from build123d import *

# Parameters (mm, degrees)
SKETCH1_R           = 1.5
BOSS_EXTRUDE1_DEPTH = 6
SKETCH2_W           = 0.5
SKETCH2_H           = 6
CUT_EXTRUDE1_DEPTH  = 0.5
FILLET1_R           = 0.5


with BuildPart() as part:
    # Sketch1 → Boss-Extrude1 (new body)
    with BuildSketch(Plane(origin=(0, 0, 0), x_dir=(1, 0, 0), z_dir=(0, 1, 0))):
        with BuildLine():
            ThreePointArc((95.828517615, 16.432423404), (96.485539703, 17.415726447), (96.511338172, 18.598053533))
            Line((96.511338172, 18.598053533), (78.7360041, 13.835167123))
            ThreePointArc((78.7360041, 13.835167123), (76.706708419, 13.046017192), (74.896318454, 11.836353292))
            Line((74.896318454, 11.836353292), (74.145485774, 11.206329867))
            ThreePointArc((74.145485774, 11.206329867), (73.602368785, 10.843430696), (72.99358008, 10.606685717))
            Line((72.99358008, 10.606685717), (44.605042506, 3))
            Line((44.605042506, 3), (0, 3))
            ThreePointArc((0, 3), (-3, 0), (0, -3))
            Line((0, -3), (44.999999999, -3))
            ThreePointArc((44.999999999, -3), (45.391578576, -2.974334584), (45.776457135, -2.897777479))
            Line((45.776457135, -2.897777479), (84.823166373, 7.564756729))
            ThreePointArc((84.823166373, 7.564756729), (85.431955077, 7.801501708), (85.975072067, 8.164400878))
            Line((85.975072067, 8.164400878), (95.828517615, 16.432423404))
        make_face()
        with Locations(Location((66.660044365, 5.803791396, 0), (0, 0, 270))):
            Circle(SKETCH1_R, mode=Mode.SUBTRACT)
        with Locations(Location((84.046709238, 10.462534208, 0), (0, 0, 270))):
            Circle(SKETCH1_R, mode=Mode.SUBTRACT)
        with Locations(Location((44.999999999, 0, 0), (0, 0, 270))):
            Circle(SKETCH1_R, mode=Mode.SUBTRACT)
        with Locations(Location((0, 0, 0), (0, 0, 270))):
            Circle(SKETCH1_R, mode=Mode.SUBTRACT)
    extrude(amount=BOSS_EXTRUDE1_DEPTH)

    # Sketch2 → Cut-Extrude1 (cut)
    with BuildSketch(Plane(origin=(1.815520398, 0, 6.775614366), x_dir=(-0.965925826289068, 0, 0.25881904510252224), z_dir=(-0.2588190451025222, 0, -0.9659258262890679))):
        with Locations((-81.167277896, 3)):
            Rectangle(SKETCH2_W, SKETCH2_H)
        with Locations((-82.567277896, 3)):
            Rectangle(SKETCH2_W, SKETCH2_H)
        with Locations((-83.967277896, 3)):
            Rectangle(SKETCH2_W, SKETCH2_H)
        with Locations((-85.367277896, 3)):
            Rectangle(SKETCH2_W, SKETCH2_H)
        with Locations((-86.767277896, 3)):
            Rectangle(SKETCH2_W, SKETCH2_H)
        with Locations((-88.167277896, 3)):
            Rectangle(SKETCH2_W, SKETCH2_H)
        with Locations((-89.567277896, 3)):
            Rectangle(SKETCH2_W, SKETCH2_H)
        with Locations((-90.967277896, 3)):
            Rectangle(SKETCH2_W, SKETCH2_H)
        with Locations((-92.367277896, 3)):
            Rectangle(SKETCH2_W, SKETCH2_H)
        with Locations((-93.767277896, 3)):
            Rectangle(SKETCH2_W, SKETCH2_H)
        with Locations((-95.167277896, 3)):
            Rectangle(SKETCH2_W, SKETCH2_H)
        with Locations((-96.567277896, 3)):
            Rectangle(SKETCH2_W, SKETCH2_H)
    extrude(amount=-CUT_EXTRUDE1_DEPTH, mode=Mode.SUBTRACT)

    # Fillet1
    # the kernel refuses this fillet: 0.5 mm, written as the material it takes off along each edge
    with BuildSketch(Plane(origin=(79.97560891, -1.25, -14.167318231), x_dir=(-0.9659258262890682, 0, 0.25881904510252096), z_dir=(0, 1, 0)), Plane(origin=(81.81086798, -1.25, -14.659074417), x_dir=(0.25881904510251386, 0, 0.9659258262890702), z_dir=(0, 1, 0)), Plane(origin=(83.163164137, -1.25, -15.02142108), x_dir=(0.2588190451025112, 0, 0.9659258262890709), z_dir=(0, 1, 0)), Plane(origin=(84.515460294, -1.25, -15.383767743), x_dir=(0.25881904510251386, 0, 0.9659258262890702), z_dir=(0, 1, 0)), Plane(origin=(85.86775645, -1.25, -15.746114406), x_dir=(0.25881904510251386, 0, 0.9659258262890702), z_dir=(0, 1, 0)), Plane(origin=(87.220052607, -1.25, -16.108461069), x_dir=(0.25881904510251214, 0, 0.9659258262890708), z_dir=(0, 1, 0)), Plane(origin=(88.572348764, -1.25, -16.470807733), x_dir=(0.25881904510251386, 0, 0.9659258262890702), z_dir=(0, 1, 0)), Plane(origin=(89.924644921, -1.25, -16.833154396), x_dir=(0.25881904510251386, 0, 0.9659258262890702), z_dir=(0, 1, 0)), Plane(origin=(91.276941078, -1.25, -17.195501059), x_dir=(0.25881904510251386, 0, 0.9659258262890702), z_dir=(0, 1, 0)), Plane(origin=(92.629237234, -1.25, -17.557847722), x_dir=(0.25881904510251563, 0, 0.9659258262890698), z_dir=(0, 1, 0)), Plane(origin=(93.981533391, -1.25, -17.920194385), x_dir=(0.25881904510251563, 0, 0.9659258262890698), z_dir=(0, 1, 0))) as fillet1_piece_1:
        with BuildLine():
            CenterArc((FILLET1_R, FILLET1_R), FILLET1_R, 180, 90)
            Line((0, FILLET1_R), (0, 0))
            Line((0, 0), (FILLET1_R, 0))
        make_face()
    extrude(amount=8.5, mode=Mode.SUBTRACT)
    with BuildSketch(Plane(origin=(95.333829548, -1.25, -18.282541048), x_dir=(0.9659258262890649, 0, -0.2588190451025338), z_dir=(0, 1, 0)), Plane(origin=(80.458571823, 7.25, -14.296727754), x_dir=(0.25881904510251386, 0, 0.9659258262890702), z_dir=(0, -1, 0)), Plane(origin=(81.327905067, 7.25, -14.529664894), x_dir=(-0.9659258262890683, 0, 0.25881904510252046), z_dir=(0, -1, 0)), Plane(origin=(82.680201224, 7.25, -14.892011557), x_dir=(-0.9659258262890675, 0, 0.2588190451025238), z_dir=(0, -1, 0)), Plane(origin=(84.03249738, 7.25, -15.254358221), x_dir=(-0.9659258262890682, 0, 0.25881904510252096), z_dir=(0, -1, 0)), Plane(origin=(85.384793537, 7.25, -15.616704884), x_dir=(-0.9659258262890675, 0, 0.2588190451025238), z_dir=(0, -1, 0)), Plane(origin=(86.737089694, 7.25, -15.979051547), x_dir=(-0.9659258262890683, 0, 0.25881904510252046), z_dir=(0, -1, 0)), Plane(origin=(88.089385851, 7.25, -16.34139821), x_dir=(-0.9659258262890683, 0, 0.25881904510252046), z_dir=(0, -1, 0)), Plane(origin=(89.441682008, 7.25, -16.703744873), x_dir=(-0.9659258262890704, 0, 0.2588190451025134), z_dir=(0, -1, 0)), Plane(origin=(90.793978164, 7.25, -17.066091536), x_dir=(-0.9659258262890683, 0, 0.25881904510252046), z_dir=(0, -1, 0)), Plane(origin=(92.146274321, 7.25, -17.428438199), x_dir=(-0.9659258262890701, 0, 0.25881904510251436), z_dir=(0, -1, 0)), Plane(origin=(93.498570478, 7.25, -17.790784863), x_dir=(-0.9659258262890682, 0, 0.25881904510252096), z_dir=(0, -1, 0)), Plane(origin=(94.850866635, 7.25, -18.153131526), x_dir=(-0.9659258262890702, 0, 0.25881904510251386), z_dir=(0, -1, 0))) as fillet1_piece_2:
        with BuildLine():
            CenterArc((FILLET1_R, -FILLET1_R), FILLET1_R, 90, 90)
            Line((0, -FILLET1_R), (0, 0))
            Line((0, 0), (FILLET1_R, 0))
        make_face()
    extrude(amount=8.5, mode=Mode.SUBTRACT)
    with BuildSketch(Plane(origin=(96.511338172, -1.657996846, -18.598053533), x_dir=(0.10403330319637054, 0, 0.9945738141666772), z_dir=(0, 1, 0))) as fillet1_piece_3:
        with BuildLine():
            CenterArc((0.584735643, -0.493805167), FILLET1_R, 80.97147389, 108.05705222)
            Line((0.090930477, -0.572268262), (0, 0))
            ThreePointArc((0, 0), (0.331599369, 0.026180497), (0.663198739, 0))
        make_face()
    extrude(amount=9.315993693, mode=Mode.SUBTRACT)


solid = part.part
Design review of the part built by this model. Coordinates are the model's own, in mm. A direction names the side the tool comes from. Coordinates: 2 decimals unless noted, no trailing zeros. Loops run counter-clockwise (first coordinate to the right, second up) from the corner with the lowest first, then second, coordinate; pieces in that order, holes last. Notation, with made-up numbers: M -25.5,13.5 L -21.5,13.5 A10 ccw -21.5,29.5 Z; hole C 11.5,-31 d2. An arc over 180 degrees is marked long. Use one line per item in the form item = value.
(1) Consider section B-B (y = 4). Give the number of separate pieces and of enclosed holes in the cut face, and give its area (3 significant figures).
Return value:
separate_pieces = 1
enclosed_holes = 4
area = 572 mm2
(2) For line 1 along Z through (x, y) = (14.5, 5.4); line 2 along X through (y, z) = (4.6, -16.75); line 3 along Z through (x, y) = (45, 4.5), list the stretches that pass through material, from the lowest coordinate up. Write a range as from..to.
Return value:
line_1 = -3..3
line_2 = 90.12..90.84, 91.4..96.14
line_3 = -3.11..-1.5, 1.5..3
(3) For faces 5 (the face through (-3, 3, 0)), 6 (the face through (23, 3, -3)), list the 3-axis set-ups (+Z, -Z, +X, -X, +Y, -Y) from which the entire face can be reached by the end or side of a thin tool; tool diameter is ignored.
Return value:
face_5 = -X, +Y, -Y
face_6 = -Z, -X, +Y, -Y
(4) Draft analysis for pull direction Z (two halves, no side actions). For faces 1 (the face through (43.536, 2.958, -0.325)), 2 (the face through (22, 3, 3)), 3 (the face through (47, 6, -3)), 4 (the face through (65.33, 2.96, -5.11)), state which applies: pulls with the +Z half, pulls with the -Z half, needs draft (parallel to the pull), parting line crosses it, or undercut.
Return value:
face_1 = undercut
face_2 = pulls with the +Z half
face_3 = needs draft
face_4 = undercut
(5) Clearance check with flat-ended pins moving along their axes: P1, Ø2.5, axis at x = 66.66, z = -5.8, coming from the -Y side (3 decimals); P2, Ø3, axis at x = 15.5, y = 1.5, coming from the -Z side. State where each tip first meets the part, or that it passes through.
Return value:
P1 = through
P2 = -3
(6) Consider section A-A (z = -0.5). Write out the cut boundary in (x, y).
Return value:
outline = M -2.96,0 L -1.41,0 L -1.41,6 L -2.96,6 Z; M 1.41,0 L 43.59,0 L 43.59,6 L 1.41,6 Z; M 46.41,0 L 58.46,0 L 58.46,6 L 46.41,6 Z
